Can you work these out from the drawing? Everything is in mm from the part's minimum corner. A direction names the side the tool comes from. Round coordinates to 2 decimals unless told otherwise and drop trailing zeros. Write each loop counter-clockwise with the first axis right and the second up, starting at its lowest first coordinate (ties: lowest second). Pieces come first, ordered by that corner, then holes. Notation, with made-up numbers: (79, -35.75) -> (89, -35.75) arc R25 cw to (89, -17.75) -> close; hole circle Ø10 at (52, 13.5). An arc over 180 degrees is marked (long way). Answer as CSV lines item,"result". Start each with the question number.
Q1. If I drill on line 1 (Z direction, x = 14.25, y = 1.6); line 2 (X direction, y = 0.8, z = 13); line 3 (Y direction, x = 12, z = 22.75), over which ranges is the centre line in solid material (lowest first)? Write a range as [from, to].
Q2. If we mould it in two halves opening along Z, with no side actions, what happens to the marked faces 1, 2, 3 and 4? For each: pulls with the +Z half, pulls with the -Z half, needs draft (parallel to the pull), parting line crosses it, or undercut.
Q3. Imagine slicing it at D-D on z = 4. Please give me the cut outline in (x, y).
Q4. Imagine slicing it at A-A on z = 13. Please give me the cut outline in (x, y).
Q5. For the marked faces 5 and 6, which set-ups out of +Z, -Z, +X, -X, +Y, -Y let a thin tool reach every point of the face, with its end or its side?
Q6. Imagine slicing it at B-B on x = 13. Please give me the cut outline in (y, z).
Q7. Will these pins go through, and if not, where does the flat tip stop? pin 1 Ø2.5 at (x, z) = (12.5, 22.5) entering from -Y; pin 2 Ø1 at (x, y) = (4, 2.5) entering from +Z; pin 3 Ø1 at (x, y) = (5, 3) entering from -Z.
Q8. Imagine slicing it at C-C on y = 1.45. Please give me the cut outline in (x, z), and give its area (3 significant figures).
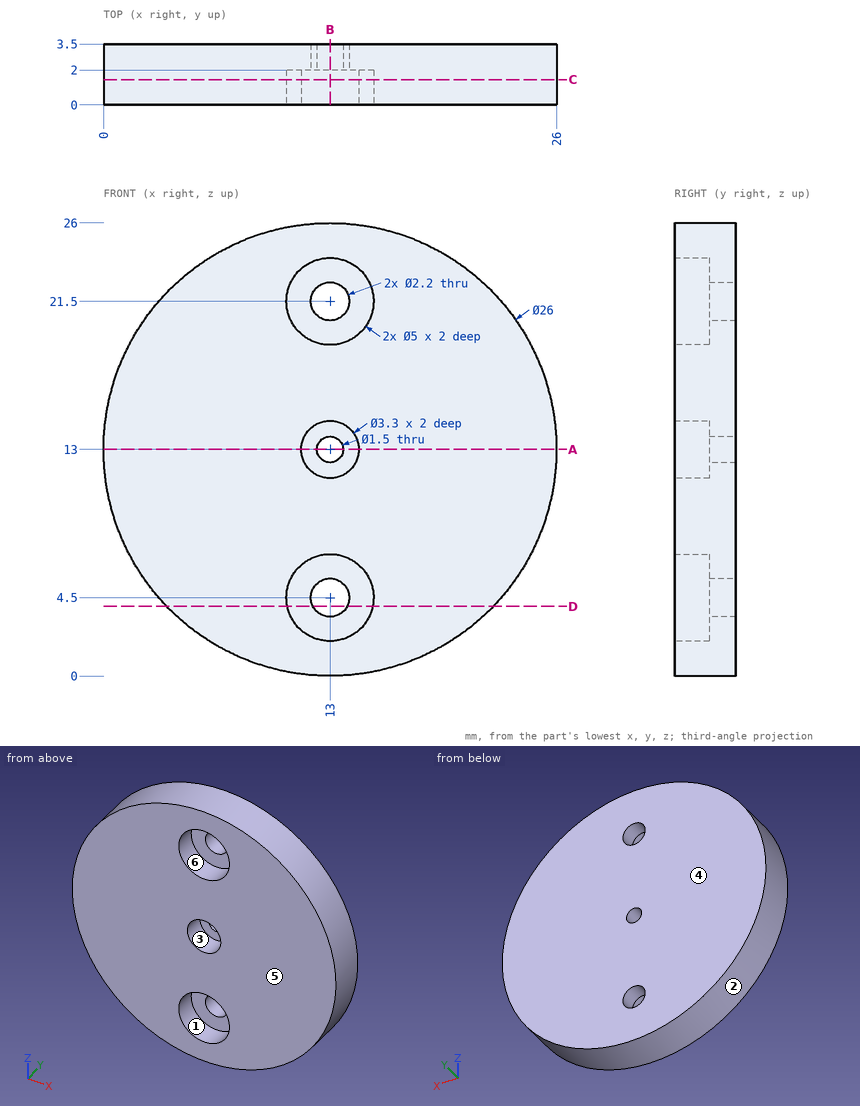
Checks:
1,line 1,"[0.06, 2.33], [6.67, 11.92], [14.08, 19.33], [23.67, 25.94]"
1,line 2,"[0, 11.35], [14.65, 26]"
1,line 3,"[2, 3.5]"
2,face 1,"undercut"
2,face 2,"parting line crosses it"
2,face 3,"undercut"
2,face 4,"needs draft"
3,outline,"(3.62, 0) -> (10.55, 0) -> (10.55, 2) -> (12.02, 2) -> (12.02, 3.5) -> (3.62, 3.5) -> close; (13.98, 2) -> (15.45, 2) -> (15.45, 0) -> (22.38, 0) -> (22.38, 3.5) -> (13.98, 3.5) -> close"
4,outline,"(0, 0) -> (11.35, 0) -> (11.35, 2) -> (12.25, 2) -> (12.25, 3.5) -> (0, 3.5) -> close; (13.75, 2) -> (14.65, 2) -> (14.65, 0) -> (26, 0) -> (26, 3.5) -> (13.75, 3.5) -> close"
5,face 5,"+Z, -Z, +X, -X, -Y"
5,face 6,"-Y"
6,outline,"(0, 0) -> (3.5, 0) -> (3.5, 3.4) -> (2, 3.4) -> (2, 2) -> (0, 2) -> close; (0, 7) -> (2, 7) -> (2, 5.6) -> (3.5, 5.6) -> (3.5, 12.25) -> (2, 12.25) -> (2, 11.35) -> (0, 11.35) -> close; (0, 14.65) -> (2, 14.65) -> (2, 13.75) -> (3.5, 13.75) -> (3.5, 20.4) -> (2, 20.4) -> (2, 19) -> (0, 19) -> close; (0, 24) -> (2, 24) -> (2, 22.6) -> (3.5, 22.6) -> (3.5, 26) -> (0, 26) -> close"
7,pin 1,"y = 2"
7,pin 2,"z = 22.84"
7,pin 3,"z = 2.38"
8,outline,"circle Ø26 at (13, 13); hole circle Ø5 at (13, 4.5); hole circle Ø5 at (13, 21.5); hole circle Ø3.3 at (13, 13)"
8,area,"483 mm^2"
